For this review, take the finished solid that the model builds, in its own axes (mm). A direction names the side the tool comes from. Give positions to 0.01 mm unless a question says otherwise; leave off trailing zeros. Loops run counter-clockwise (first coordinate to the right, second up) from the corner with the lowest first, then second, coordinate; pieces in that order, holes last. Notation, with made-up numbers: (-19.5, -23.5) - (-13.5, -23.5) arc R17 cw to (-13.5, 2.5) - close; hole circle Ø7 at (53, 39). An arc over 180 degrees is marked (long way). Answer in a Markdown table with one row per item.
```python
from build123d import *

# Parameters (mm, degrees)
F0_W     = 12.7
F0_H     = 19.05
F1_DEPTH = 19.05
F3_DEPTH = 19.05
F5_DEPTH = 19.05


with BuildPart() as f1:
    # F0 (on Front) → F1 (new body)
    with BuildSketch(Plane.XZ):
        Polygon((-21.9277606558, 43.1296415627), (-40.9777606558, 43.1296415627), (-61.0902286349, 23.0171667248), (-73.7902286349, 23.0171667248), (-73.7902286349, 3.9671667248), (-61.0902286349, 3.9671667248), (-40.9777637411, -16.1453046837), (-21.9277637411, -16.1453046837), (-1.8152923326, 3.9671667248), (10.8847076674, 3.9671667248), (10.8847076674, 23.0171667248), (-1.8152923326, 23.0171667248), align=None)
        Polygon((-53.0427621984, 10.3171667248), (-9.8627621984, 10.3171667248), (-9.8627621984, 2.6971667248), (-20.639071289, -8.0791388752), (-42.2664548532, -8.0791406205), (-53.0427621984, 2.6971667248), align=None, mode=Mode.SUBTRACT)
        Polygon((-9.8627621984, 16.6671667248), (-53.0427621984, 16.6671667248), (-53.0427621984, 24.2871667248), (-42.2664531079, 35.0634723248), (-20.6390695437, 35.0634740701), (-9.8627621984, 24.2871667248), align=None, mode=Mode.SUBTRACT)
        with Locations((-80.1402286349, 13.4921667248)):
            Rectangle(F0_W, F0_H)
        with Locations((17.2347076674, 13.4921667248)):
            Rectangle(F0_W, F0_H)
    extrude(amount=F1_DEPTH)

    # F2 (on face) → F3 (join)
    with BuildSketch(Plane(origin=(0, 0, 3.9671667248), x_dir=(1, 0, 0), z_dir=(0, 0, -1))):
        with BuildLine():
            Line((10.8847076674, 19.05), (23.5847076674, 19.05))
            Line((23.5847076674, 19.05), (23.5847076674, 31.75))
            add(Edge.make_bspline(
                [(10.8847076674, 19.05), (13.2814331351, 20.2980463011), (18.3522044059, 22.9385478577), (21.7780861226, 28.7076780967), (23.5847076674, 31.75)],
                knots=[0, 0, 0, 0, 0.4726550143, 1, 1, 1, 1], degree=3))
        make_face()
    extrude(amount=-F3_DEPTH)

    # F4 (on face) → F5 (join)
    with BuildSketch(Plane(origin=(0, 0, 3.9671667248), x_dir=(1, 0, 0), z_dir=(0, 0, -1))):
        with BuildLine():
            Line((-86.4902286349, 31.75), (-86.4902286349, 19.05))
            Line((-86.4902286349, 19.05), (-73.7902286349, 19.05))
            add(Edge.make_bspline(
                [(-73.7902286349, 19.05), (-76.7799525344, 20.4645934924), (-82.6711867803, 23.2520420685), (-85.2299862455, 28.9457660543), (-86.4902286349, 31.75)],
                knots=[0, 0, 0, 0, 0.5074868482, 1, 1, 1, 1], degree=3))
        make_face()
    extrude(amount=-F5_DEPTH)


solid = f1.part
```
1. We need section B-B, the plane y = -7.5. Give the boundary of the cut face in (x, z), and give its area (3 significant figures).
Values:
| item | result |
|---|---|
| outline | (-86.49, 3.97) - (-61.09, 3.97) - (-40.98, -16.15) - (-21.93, -16.15) - (-1.82, 3.97) - (23.58, 3.97) - (23.58, 23.02) - (-1.82, 23.02) - (-21.93, 43.13) - (-40.98, 43.13) - (-61.09, 23.02) - (-86.49, 23.02) - close; hole (-53.04, 2.7) - (-42.27, -8.08) - (-20.64, -8.08) - (-9.86, 2.7) - (-9.86, 10.32) - (-53.04, 10.32) - close; hole (-53.04, 16.67) - (-9.86, 16.67) - (-9.86, 24.29) - (-20.64, 35.06) - (-42.27, 35.06) - (-53.04, 24.29) - close |
| area | 2,320 mm^2 |
2. Mouldability with a two-part tool opening along Z and no side actions: class faces 1 (the face through (-86.49, -16, 13)), 2 (the face through (-47.73, -9.39, 29.6)), 3 (the face through (-32, -9, -16.145)) as released by +Z, released by -Z, zero draft, split by the parting line, or undercut.
Values:
| item | result |
|---|---|
| face 1 | zero draft |
| face 2 | undercut |
| face 3 | released by -Z |
3. Clearance check with flat-ended pins moving along their axes: pin 1 (18 mm diameter, centred on x = -12, z = 20.5, fed in from -Y); pin 2 (10 mm diameter, centred on x = -63.5, y = -17, fed in from +Z); pin 3 (7.5 mm diameter, centred on x = 15, y = -9, fed in from -Z). State where each tip first meets the part, or that it passes through.
Values:
| item | result |
|---|---|
| pin 1 | stops at y = -19.05 |
| pin 2 | stops at z = 25.61 |
| pin 3 | stops at z = 3.97 |
4. We need section C-C, the plane z = -3.5. Give the boundary of the cut face in (x, y), and give its area (3 significant figures).
Values:
| item | result |
|---|---|
| outline | (-53.62, -19.05) - (-46.85, -19.05) - (-46.85, 0) - (-53.62, 0) - close; (-16.06, -19.05) - (-9.28, -19.05) - (-9.28, 0) - (-16.06, 0) - close |
| area | 258 mm^2 |
5. We need section A-A, the plane x = -38.5. Give the boundary of the cut face in (y, z).
Values:
| item | result |
|---|---|
| outline | (-19.05, -16.15) - (0, -16.15) - (0, -8.08) - (-19.05, -8.08) - close; (-19.05, 10.32) - (0, 10.32) - (0, 16.67) - (-19.05, 16.67) - close; (-19.05, 35.06) - (0, 35.06) - (0, 43.13) - (-19.05, 43.13) - close |
6. For faces 4 (the face through (-32, -9, 35.063)), 5 (the face through (-32, -19.05, 11)), 6 (the face through (-74, -9, 3.967)), list the 3-axis set-ups (+Z, -Z, +X, -X, +Y, -Y) from which the entire face can be reached by the end or side of a thin tool; tool diameter is ignored.
Values:
| item | result |
|---|---|
| face 4 | +Y, -Y |
| face 5 | +Z, -Z, -Y |
| face 6 | -Z, -X, +Y, -Y |
7. We need section D-D, the plane z = 39.5. Give the boundary of the cut face in (x, y).
Values:
| item | result |
|---|---|
| outline | (-44.61, -19.05) - (-18.3, -19.05) - (-18.3, 0) - (-44.61, 0) - close |
8. Wall thickness on line 1 (Z direction, x = -38, y = -18); line 2 (X direction, y = -3.5, z = 7); line 3 (Z direction, x = -18, y = -17): over which ranges is each line inside the solid? List them lowest first. Write a range as [from, to].
Values:
| item | result |
|---|---|
| line 1 | z = [-16.15, -8.08], [10.32, 16.67], [35.06, 43.13] |
| line 2 | x = [-86.49, -53.04], [-9.86, 23.58] |
| line 3 | z = [-12.22, -5.44], [10.32, 16.67], [32.42, 39.2] |
